```python
from build123d import *

# Parameters (mm, degrees)
SKETCH1_R           = 14.9
SKETCH1_R_2         = 1.6000000000000003
SKETCH1_R_3         = 1.6000000000006653
SKETCH1_R_4         = 1.6000000000009684
SKETCH1_R_5         = 2.5
BOSS_EXTRUDE1_DEPTH = 5
CUT_EXTRUDE1_DEPTH  = 3.5
CUT_EXTRUDE2_DEPTH  = 22.656869579881576
FILLET1_R           = 10
FILLET2_R           = 2
SKETCH6_R           = 2.4999999999999956
BOSS_EXTRUDE2_DEPTH = 5


with BuildPart() as part:
    # Sketch1 → Boss-Extrude1 (new body)
    with BuildSketch(Plane.XY):
        Circle(SKETCH1_R)
        with Locations((0, 12)):
            Circle(SKETCH1_R_2, mode=Mode.SUBTRACT)
        with Locations((10.392304845414033, -5.99999999999955)):
            Circle(SKETCH1_R_3, mode=Mode.SUBTRACT)
        with Locations((-10.3923048454125, -6.000000000000447)):
            Circle(SKETCH1_R_4, mode=Mode.SUBTRACT)
        Circle(SKETCH1_R_5, mode=Mode.SUBTRACT)
    extrude(amount=BOSS_EXTRUDE1_DEPTH)

    # Sketch2 → Cut-Extrude1 (cut)
    with BuildSketch(Plane.XY.offset(5)):
        Polygon((13.142304845413232, -7.5877132402708165), (13.142304845413246, -4.412286759728591), (10.392304845413825, -2.824573519457418), (7.642304845414409, -4.41228675972855), (7.64230484541441, -7.587713240270817), (10.39230484541382, -9.17542648054195), align=None)
        Polygon((1.342e-14, 15.175426480542264), (-2.749999999999405, 13.58771324027113), (-2.7499999999994076, 10.412286759728874), (9e-15, 8.824573519457736), (2.7499999999994245, 10.41228675972887), (2.7499999999994267, 13.58771324027113), align=None)
        Polygon((-13.14230484541212, -7.587713240271449), (-10.3923048454127, -9.175426480542583), (-7.642304845413332, -7.587713240271399), (-7.642304845413293, -4.412286759729188), (-10.392304845412706, -2.8245735194580552), (-13.142304845412118, -4.4122867597291835), align=None)
    extrude(amount=-CUT_EXTRUDE1_DEPTH, mode=Mode.SUBTRACT)

    # Sketch5 → Cut-Extrude2 (cut, through all)
    with BuildSketch(Plane.XY.offset(5)):
        with BuildLine():
            Line((4, 14.353048456686821), (4, 7.613146524269713))
            ThreePointArc((4, 7.613146524269714), (7.360706487831178, 4.447471191587419), (8.600000000000001, 0))
            ThreePointArc((8.600000000000001, 0), (8.598294404056443, -0.17126979059858147), (8.593178292750771, -0.3424716469971399))
            Line((8.593178292750771, -0.3424716469971399), (14.430104585239802, -3.712422613205722))
            ThreePointArc((14.430104585239803, -3.712422613205722), (12.903778516388154, 7.44999999999997), (4.000000000000001, 14.353048456686825))
        make_face()
        with BuildLine():
            Line((-14.43010458523985, -3.712422613205522), (-8.593178292750776, -0.3424716469970228))
            ThreePointArc((-8.593178292750778, -0.3424716469970228), (-7.447818472546155, 4.300000000000037), (-4.000000000000002, 7.613146524269715))
            Line((-4, 7.613146524269713), (-4, 14.353048456686821))
            ThreePointArc((-3.9999999999999996, 14.35304845668682), (-12.903778516388101, 7.450000000000059), (-14.43010458523985, -3.712422613205523))
        make_face()
        with BuildLine():
            ThreePointArc((4.593178292750738, -7.270674877272635), (-6.195e-14, -8.6), (-4.593178292750841, -7.270674877272569))
            Line((-4.59317829275084, -7.270674877272568), (-10.43010458523992, -10.640625843481063))
            ThreePointArc((-10.430104585239919, -10.640625843481068), (-1.0303e-13, -14.899999999999999), (10.430104585239771, -10.640625843481217))
            Line((10.430104585239768, -10.640625843481212), (4.593178292750737, -7.270674877272635))
        make_face()
    extrude(amount=-CUT_EXTRUDE2_DEPTH, mode=Mode.SUBTRACT)

    # Fillet1
    fillet1_edges = [part.edges().sort_by_distance(p)[0] for p in [
        (4.593178292750738, -7.270674877272635, 2.5),
        (-4.593178292750841, -7.270674877272569, 2.5),
        (-4.000000000000001, 7.613146524269714, 2.5),
        (-8.593178292750778, -0.3424716469970228, 2.5),
        (4.000000000000001, 7.613146524269715, 2.5),
        (8.593178292750771, -0.3424716469971399, 2.5),
    ]]
    fillet(fillet1_edges, radius=FILLET1_R)

    # Fillet2
    fillet2_edges = [part.edges().sort_by_distance(p)[0] for p in [
        (10.430104585239771, -10.640625843481214, 2.5),
        (-10.43010458523992, -10.640625843481068, 2.5),
        (-14.43010458523985, -3.7124226132055225, 2.5),
        (-4, 14.353048456686821, 2.5),
        (4, 14.353048456686823, 2.5),
        (14.430104585239803, -3.712422613205722, 2.5),
    ]]
    fillet(fillet2_edges, radius=FILLET2_R)

    # Sketch6 → Boss-Extrude2 (add)
    with BuildSketch(Plane.XY.offset(5)):
        with BuildLine():
            ThreePointArc((6.02817063707193, 5.259387680171888), (4.855499076696584, 4.968349486507053), (3.914637171074405, 4.2102988989907315))
            ThreePointArc((3.914637171074405, 4.2102988989907315), (3.5015459862118337, 4.559624623414058), (3.0574479574494795, 4.868574019924936))
            ThreePointArc((3.0574479574494795, 4.868574019924936), (3.547016405974829, 5.9731936616538555), (3.5255692044436264, 7.181250711726956))
            ThreePointArc((3.5255692044436264, 7.181250711726956), (3.3385186822805317, 7.270095804600103), (3.1492312822635022, 7.354069780115842))
            ThreePointArc((3.1492312822635022, 7.354069780115842), (2.2189674537840838, 6.583050306880795), (1.7001859911750001, 5.491845645628829))
            ThreePointArc((1.7001859911750001, 5.491845645628829), (1.1764369425261552, 5.627343700207033), (0.6422703249581851, 5.713010574966424))
            ThreePointArc((0.6422703249581851, 5.713010574966424), (0.6040797553307691, 6.9206542720378605), (0.06060018449448659, 7.999770472809791))
            ThreePointArc((0.06060018449448659, 7.999770472809791), (-0.1464749537974085, 7.998658955594381), (-0.3534519507842858, 7.992188168360838))
            ThreePointArc((-0.3534519507842858, 7.992188168360838), (-0.8570578872002823, 6.893897278163069), (-0.8510078756894319, 5.685665009083339))
            ThreePointArc((-0.8510078756894319, 5.685665009083339), (-1.3816798656790947, 5.580498342332617), (-1.9001168223196914, 5.425915320159152))
            ThreePointArc((-1.9001168223196914, 5.425915320159152), (-2.4585022994085572, 6.497394427590124), (-3.4163714452062757, 7.233837581006314))
            ThreePointArc((-3.4163714452062757, 7.233837581006314), (-3.6024574288783424, 7.14298960331872), (-3.7861296901755246, 7.047355672106486))
            ThreePointArc((-3.7861296901755246, 7.047355672106486), (-3.7633324024994224, 5.8393233454034945), (-3.233649195846893, 4.753368687383592))
            ThreePointArc((-3.233649195846893, 4.753368687383592), (-3.6661380312950715, 4.428366847438451), (-4.066162529533613, 4.064150991709943))
            ThreePointArc((-4.066162529533613, 4.064150991709943), (-5.034147822198015, 4.787245931444861), (-6.216688811137787, 5.035154439088672))
            ThreePointArc((-6.216688811137787, 5.035154439088672), (-6.344929028928957, 4.8725635570872505), (-6.468918010594077, 4.7067079548461095))
            ThreePointArc((-6.468918010594077, 4.7067079548461095), (-5.9242327812405176, 3.628199809485637), (-4.975826634662063, 2.879609400906265))
            ThreePointArc((-4.975826634662063, 2.879609400906265), (-5.224472597580759, 2.3991429880538346), (-5.426854879562582, 1.897431715811644))
            ThreePointArc((-5.426854879562582, 1.897431715811644), (-6.61271862902979, 2.1289246668585444), (-7.785714715338611, 1.8391972083928103))
            ThreePointArc((-7.785714715338611, 1.8391972083928103), (-7.83070961935227, 1.637066540304308), (-7.8704577829414815, 1.4338390031436454))
            ThreePointArc((-7.8704577829414815, 1.4338390031436454), (-6.911766201709898, 0.6984668043486959), (-5.7324805839734525, 0.43550815648784985))
            ThreePointArc((-5.7324805839734525, 0.43550815648784985), (-5.748036291964011, -0.1052605636725878), (-5.712692064686818, -0.6450971818759339))
            ThreePointArc((-5.712692064686818, -0.6450971818759339), (-6.881559411710404, -0.9510562375466041), (-7.812684334641904, -1.7210355856986488))
            ThreePointArc((-7.812684334641904, -1.7210355856986488), (-7.765522132311889, -1.9226715820894416), (-7.713156866547124, -2.1230193480128765))
            ThreePointArc((-7.713156866547124, -2.1230193480128765), (-6.530339558681069, -2.3696061175227916), (-5.353746449368295, -2.0948508194800826))
            ThreePointArc((-5.353746449368295, -2.0948508194800826), (-5.1331309036849415, -2.5888159698276345), (-4.867060524829484, -3.059856671095323))
            ThreePointArc((-4.867060524829484, -3.059856671095323), (-5.78742295611416, -3.842668790166433), (-6.292256005183971, -4.940396174926289))
            ThreePointArc((-6.292256005183971, -4.940396174926289), (-6.162277749088176, -5.101601017630917), (-6.028170637071975, -5.259387680171835))
            ThreePointArc((-6.028170637071975, -5.259387680171835), (-4.855499076696629, -4.968349486507008), (-3.9146371710744448, -4.210298898990695))
            ThreePointArc((-3.9146371710744448, -4.210298898990695), (-3.5015459862118763, -4.559624623414024), (-3.0574479574495212, -4.868574019924903))
            ThreePointArc((-3.0574479574495212, -4.868574019924903), (-3.5470164059748766, -5.973193661653813), (-3.525569204443685, -7.1812507117269115))
            ThreePointArc((-3.525569204443685, -7.1812507117269115), (-3.338518682280587, -7.2700958046000626), (-3.1492312822635578, -7.35406978011581))
            ThreePointArc((-3.1492312822635578, -7.35406978011581), (-2.218967453784133, -6.583050306880769), (-1.700185991175043, -5.491845645628806))
            ThreePointArc((-1.700185991175043, -5.491845645628806), (-1.176436942526202, -5.627343700207011), (-0.6422703249582338, -5.713010574966406))
            ThreePointArc((-0.6422703249582338, -5.713010574966406), (-0.6040797553308295, -6.920654272037842), (-0.06060018449455164, -7.999770472809773))
            ThreePointArc((-0.06060018449455164, -7.999770472809773), (0.14647495379734404, -7.998658955594365), (0.35345195078422115, -7.9921881683608245))
            ThreePointArc((0.35345195078422115, -7.9921881683608245), (0.8570578872002264, -6.893897278163062), (0.8510078756893855, -5.6856650090833325))
            ThreePointArc((0.8510078756893855, -5.6856650090833325), (1.3816798656790477, -5.580498342332614), (1.900116822319644, -5.425915320159157))
            ThreePointArc((1.900116822319644, -5.425915320159157), (2.458502299408505, -6.497394427590132), (3.416371445206218, -7.23383758100633))
            ThreePointArc((3.416371445206218, -7.23383758100633), (3.6024574288782856, -7.142989603318738), (3.7861296901754686, -7.047355672106509))
            ThreePointArc((3.7861296901754686, -7.047355672106509), (3.7633324024993775, -5.839323345403511), (3.2336491958468514, -4.753368687383601))
            ThreePointArc((3.2336491958468514, -4.753368687383601), (3.6661380312950302, -4.428366847438464), (4.066162529533574, -4.064150991709959))
            ThreePointArc((4.066162529533574, -4.064150991709959), (5.034147822197974, -4.7872459314448825), (6.216688811137743, -5.035154439088707))
            ThreePointArc((6.216688811137743, -5.035154439088707), (6.344929028928913, -4.872563557087289), (6.468918010594035, -4.706707954846148))
            ThreePointArc((6.468918010594035, -4.706707954846148), (5.924232781240482, -3.628199809485669), (4.975826634662032, -2.8796094009062863))
            ThreePointArc((4.975826634662032, -2.8796094009062863), (5.224472597580731, -2.3991429880538595), (5.426854879562554, -1.8974317158116716))
            ThreePointArc((5.426854879562554, -1.8974317158116716), (6.6127186290297635, -2.128924666858581), (7.7857147153385915, -1.8391972083928554))
            ThreePointArc((7.7857147153385915, -1.8391972083928554), (7.830709619352263, -1.6370665403042963), (7.870457782941487, -1.433839003143578))
            ThreePointArc((7.870457782941487, -1.433839003143578), (6.911766201709897, -0.6984668043486324), (5.732480583973447, -0.435508156487793))
            ThreePointArc((5.732480583973447, -0.435508156487793), (5.748036291964002, 0.10526056367264261), (5.7126920646868085, 0.6450971818759847))
            ThreePointArc((5.7126920646868085, 0.6450971818759847), (6.881559411710389, 0.9510562375466631), (7.81268433464188, 1.7210355856987143))
            ThreePointArc((7.81268433464188, 1.7210355856987143), (7.7655221323118635, 1.9226715820895108), (7.713156866547099, 2.123019348012948))
            ThreePointArc((7.713156866547099, 2.123019348012948), (6.530339558681042, 2.3696061175228524), (5.35374644936827, 2.094850819480135))
            ThreePointArc((5.35374644936827, 2.094850819480135), (5.133130903684914, 2.5888159698276865), (4.8670605248294505, 3.059856671095373))
            ThreePointArc((4.8670605248294505, 3.059856671095373), (5.787422956114117, 3.8426687901664893), (6.29225600518392, 4.940396174926349))
            ThreePointArc((6.29225600518392, 4.940396174926349), (6.162277749088128, 5.101601017630973), (6.02817063707193, 5.259387680171888))
        make_face()
        Circle(SKETCH6_R, mode=Mode.SUBTRACT)
    extrude(amount=BOSS_EXTRUDE2_DEPTH)


solid = part.part
```
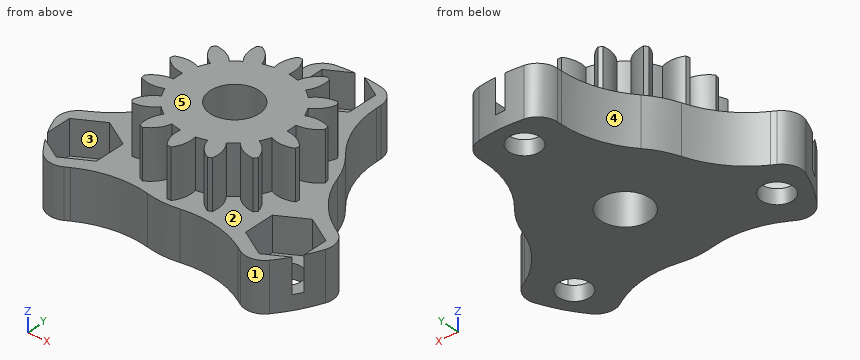
Design review of the part built by this model. Coordinates are the model's own, in mm. Face numbers are marked on the shaded views. A direction names the side the tool comes from. Coordinates: 2 decimals unless noted, no trailing zeros. Loops run counter-clockwise (first coordinate to the right, second up) from the corner with the lowest first, then second, coordinate; pieces in that order, holes last.
Q1. For pin 1 (4 mm diameter, centred on y = -1, z = 8, fed in from -X); pin 2 (6 mm diameter, centred on y = 5.5, z = 6.5, fed in from +X); pin 3 (3.5 mm diameter, centred on y = 12.5, z = 3.5, fed in from -X), all flat-tipped, find the tip position at first contact; note any pin that passes through.
Reported:
pin 1: stops at x = -7.81
pin 2: stops at x = 8.1
pin 3: stops at x = -4.11
Q2. To check wall thickness, follow line 1 (Y direction, x = 0, z = 0.3); line 2 (X direction, y = -4.5, z = 4.75); line 3 (Y direction, x = 0, z = 8.5). State the ranges of each line that lie inside material, in increasing order.
Reported:
line 1: y = -8.6 to -2.5, 2.5 to 10.4, 13.6 to 14.9
line 2: x = -14.03 to -13.14, -7.64 to 7.64, 13.14 to 14.03
line 3: y = -8 to -2.5, 2.5 to 8
Q3. Tool access review of the marked faces 1 and 2: name each direction out of +Z, -Z, +X, -X, +Y, -Y from which nothing blocks a thin tool from reaching the whole face with its end or side.
Reported:
face 1: +Z, -Z, -Y
face 2: +Z
Q4. The part is to be moulded in two halves that separate along Y. For the marked faces 3, 4 and 5, say which applies: +Y half, -Y half, draft (parallel to the pull), parting line (faces both ways), or undercut.
Reported:
face 3: undercut
face 4: +Y half
face 5: draft
Q5. We need section A-A on y = 0. State the section outline as (x, z) points.
Reported:
outline: (-9.61, 0) - (-2.5, 0) - (-2.5, 10) - (-5.75, 10) - (-5.75, 5) - (-9.61, 5) - close; (2.5, 0) - (9.61, 0) - (9.61, 5) - (5.75, 5) - (5.75, 10) - (2.5, 10) - close
